Geometry: final body of the model. Coordinates: model frame, mm. A direction names the side the tool comes from. Round coordinates to 2 decimals unless told otherwise and drop trailing zeros. Loops run counter-clockwise (first coordinate to the right, second up) from the corner with the lowest first, then second, coordinate; pieces in that order, holes last. Notation, with made-up numbers: (-17.75, -38) -> (31.25, -38) arc R19 cw to (31.25, -1) -> close; hole circle Ø9 at (87.5, 70). An arc over 180 degrees is marked (long way). Answer in a Markdown table with one row per item.
```python
from build123d import *

# Parameters (mm, degrees)
F1_DEPTH = 12.7
F2_W     = 19.05
F2_H     = 50.8
F3_DEPTH = 15.875
F5_DEPTH = 19.05
F6_R     = 9.525
F7_DEPTH = 19.05


with BuildPart() as f1:
    # F0 (on Top) → F1 (new body)
    with BuildSketch(Plane.XY):
        with BuildLine():
            Line((36.467142, 20.915313), (-39.732858, 20.915313))
            Line((-39.732858, 20.915313), (-39.732858, 5.040313))
            ThreePointArc((-39.732858, 5.040313), (-32.997666, 2.250505), (-30.207858, -4.484687))
            ThreePointArc((-30.207858, -4.484687), (-32.997666, -11.219879), (-39.732858, -14.009687))
            Line((-39.732858, -14.009687), (-39.732858, -29.884687))
            Line((-39.732858, -29.884687), (36.467142, -29.884687))
            Line((36.467142, -29.884687), (36.467142, -14.009687))
            ThreePointArc((36.467142, -14.009687), (26.942142, -4.484687), (36.467142, 5.040313))
            Line((36.467142, 5.040313), (36.467142, 20.915313))
        make_face()
        with BuildLine():
            Line((-39.732858, 5.040313), (-39.732858, 20.915313))
            ThreePointArc((-39.732858, 20.915313), (-65.132858, -4.484687), (-39.732858, -29.884687))
            Line((-39.732858, -29.884687), (-39.732858, -14.009687))
            ThreePointArc((-39.732858, -14.009687), (-49.257858, -4.484687), (-39.732858, 5.040313))
        make_face()
        with BuildLine():
            ThreePointArc((36.467142, -29.884687), (61.867142, -4.484687), (36.467142, 20.915313))
            Line((36.467142, 20.915313), (36.467142, 5.040313))
            ThreePointArc((36.467142, 5.040313), (43.202334, 2.250505), (45.992142, -4.484687))
            ThreePointArc((45.992142, -4.484687), (43.202334, -11.219879), (36.467142, -14.009687))
            Line((36.467142, -14.009687), (36.467142, -29.884687))
        make_face()
    extrude(amount=F1_DEPTH)

    # F2 (on face) → F3 (join)
    with BuildSketch(Plane.XY.offset(12.7)):
        with Locations((-1.632858, -4.484687)):
            Rectangle(F2_W, F2_H)
    extrude(amount=F3_DEPTH)

    # F4 (on face) → F5 (join)
    with BuildSketch(Plane(origin=(-11.157858, 0, 0), x_dir=(0, -1, 0), z_dir=(-1, 0, 0))):
        with BuildLine():
            Line((-20.915313, 28.575), (29.884687, 28.575))
            ThreePointArc((29.884687, 28.575), (4.484687, 53.975), (-20.915313, 28.575))
        make_face()
    extrude(amount=-F5_DEPTH)

    # F6 (on face) → F7 (cut)
    with BuildSketch(Plane(origin=(-11.157858, 0, 0), x_dir=(0, -1, 0), z_dir=(-1, 0, 0))):
        with Locations((4.484687, 28.575)):
            Circle(F6_R)
    extrude(amount=-F7_DEPTH, mode=Mode.SUBTRACT)


solid = f1.part
```
Item 1: Ray query, L1, parallel to Z at x = 16, y = 12; L2, parallel to X at y = 2, z = 4; L3, parallel to X at y = 2.5, z = 6.5. Return the intervals inside material, ascending.
Ans:
| item | result |
|---|---|
| L1 | 0 to 12.7 |
| L2 | -64.29 to -46.71, -32.76 to 29.49, 43.44 to 61.03 |
| L3 | -64.15 to -46.21, -33.26 to 29.99, 42.94 to 60.89 |
Item 2: Section query D-D, the plane z = 26.5. Output: boundary loops of the cut face in (x, y), and give its area (3 significant figures).
Ans:
| item | result |
|---|---|
| outline | (-11.16, -29.88) -> (7.89, -29.88) -> (7.89, -13.78) -> (-11.16, -13.78) -> close; (-11.16, 4.81) -> (7.89, 4.81) -> (7.89, 20.92) -> (-11.16, 20.92) -> close |
| area | 614 mm2 |
Item 3: Section query A-A, the plane z = 10.5. Output: boundary loops of the cut face in (x, y) (3 decimals).
Ans:
| item | result |
|---|---|
| outline | (-39.733, -29.885) -> (36.467, -29.885) arc R25.4 ccw to (36.467, 20.915) -> (-39.733, 20.915) arc R25.4 ccw to start; hole circle Ø19.05 at (-39.733, -4.485); hole circle Ø19.05 at (36.467, -4.485) |
Item 4: Set-up query: faces 4 (the flat face through (7.892, -10, 38)), 5 (the flat face through (-3, -4, 0)), 6 (the flat face through (-11.158, -10, 38)). Return all of +Z, -Z, +X, -X, +Y, -Y with unobstructed straight access to the full face (end or side cutting, diameter ignored); none if empty.
Ans:
| item | result |
|---|---|
| face 4 | +Z, +X, +Y, -Y |
| face 5 | -Z, +X, -X, +Y, -Y |
| face 6 | +Z, -X, +Y, -Y |
Item 5: Mould query, pull axis Z, two halves, no side actions, for faces 1 (the cylindrical face through (-1.77, 2.54, 35.01)), 2 (the cylindrical face through (-65.127, -3.926, 6.261)), 3 (the flat face through (29, 2, 12.7)). Classes: released by +Z, released by -Z, zero draft, split by the parting line, or undercut.
Ans:
| item | result |
|---|---|
| face 1 | undercut |
| face 2 | zero draft |
| face 3 | released by +Z |
Item 6: Section query C-C, the plane y = 0. Output: boundary loops of the cut face in (x, z), and give its area (3 significant figures).
Ans:
| item | result |
|---|---|
| outline | (-64.73, 0) -> (-48.14, 0) -> (-48.14, 12.7) -> (-64.73, 12.7) -> close; (-31.33, 0) -> (28.06, 0) -> (28.06, 12.7) -> (7.89, 12.7) -> (7.89, 20.17) -> (-11.16, 20.17) -> (-11.16, 12.7) -> (-31.33, 12.7) -> close; (-11.16, 36.98) -> (7.89, 36.98) -> (7.89, 53.58) -> (-11.16, 53.58) -> close; (44.87, 0) -> (61.47, 0) -> (61.47, 12.7) -> (44.87, 12.7) -> close |
| area | 1,630 mm2 |
Item 7: First-contact query: P1, Ø12.5, axis at y = -15, z = 37.5, coming from the +X side; P2, Ø22, axis at y = -4.48, z = 28.58, coming from the -X side; P3, Ø3, axis at x = -44, z = 8.5, coming from the +Y side. Flat tips, straight axial feed; report the tip coordinate or a pass-through.
Ans:
| item | result |
|---|---|
| P1 | x = 7.89 |
| P2 | x = -11.16 |
| P3 | y = 20.76 |
Item 8: Section query B-B, the plane x = -9. Output: boundary loops of the cut face in (y, z) (3 decimals).
Ans:
| item | result |
|---|---|
| outline | (-29.885, 0) -> (20.915, 0) -> (20.915, 28.575) arc R25.4 ccw to (-29.885, 28.575) -> close; hole circle Ø19.05 at (-4.485, 28.575) |
